Geometry: final body of the model. Coordinates: model frame, mm. A direction names the side the tool comes from. Give positions to 0.01 mm unless a question says otherwise; leave off trailing zeros. Loops run counter-clockwise (first coordinate to the right, second up) from the corner with the lowest first, then second, coordinate; pieces in that order, holes last. Notation, with made-up numbers: (-23, 8.25) -> (4, 8.25) arc R11 cw to (4, 29.25) -> close; hole circle Ø3 at (-38, 7). An arc over 180 degrees is marked (long way). Answer in a Markdown table with one row per item. Add a question column.
1) Section query B-B (y = 4.5). Return the cut outline in (x, z), plus the area to 3 significant figures.
2) Line query: line 1 (Z direction, x = 272, y = 6.75); line 2 (Y direction, x = 129, z = 2.5). Output: solid intervals per line, ascending. Write a range as from..to.
3) Access query for faces 1 (the flat face through (192, 9, 0)), 2 (the flat face through (192, 0, 7)). Directions: +Z, -Z, +X, -X, +Y, -Y. A direction counts if a zero-diameter tool reaches every point of the face in a straight line with its end or side. Return the directions, or none.
4) Section query A-A (x = 66.5). Return the cut outline in (y, z), plus the area to 3 significant figures.
5) First-contact query: P1, Ø4, axis at x = 17.145, z = 6.096, coming from the +Y side; P2, Ø4.5, axis at x = 258.445, y = 9.398, coming from the +Z side. Flat tips, straight axial feed; report the tip coordinate or a pass-through.
```python
from build123d import *

# Parameters (mm, degrees)
SKETCH1_W                    = 389.89
SKETCH1_H                    = 15.24
BASE_FLANGE1_DEPTH           = 1.524
EDGE_FLANGE1_STRIP_W         = 6.4008
EDGE_FLANGE1_STRIP_H         = 1.524
EDGE_FLANGE1_STRIP_CUT_DEPTH = 389.89
EDGE_FLANGE1_DEPTH           = 389.89
SKETCH9_R                    = 2.032
CUT_EXTRUDE1_DEPTH           = 2.54
SKETCH10_R                   = 1.778
CUT_EXTRUDE2_DEPTH           = 2.54


# Sheet-metal steps are written as plain solids
with BuildPart() as part:
    # Sketch1 → Base-Flange1 (new body)
    with BuildSketch(Plane.XY):
        with Locations((194.945, 7.62)):
            Rectangle(SKETCH1_W, SKETCH1_H)
    extrude(amount=-BASE_FLANGE1_DEPTH)

    # Edge-Flange1 strip (across the edge) → Edge-Flange1 strip cut (cut)
    with BuildSketch(Plane.YZ):
        with Locations((-1.524, -0.762)):
            Rectangle(EDGE_FLANGE1_STRIP_W, EDGE_FLANGE1_STRIP_H)
    extrude(amount=EDGE_FLANGE1_STRIP_CUT_DEPTH, mode=Mode.SUBTRACT)

    # Edge-Flange1 section (across the edge) → Edge-Flange1 (add)
    with BuildSketch(Plane.YZ):
        with BuildLine():
            Line((0, 0.1524), (0, 13.716))
            Line((0, 13.716), (1.524, 13.716))
            Line((1.524, 13.716), (1.524, 0.1524))
            ThreePointArc((1.524, 0.1524), (1.568636927, 0.044636927), (1.6764, 0))
            Line((1.6764, 0), (1.6764, -1.524))
            ThreePointArc((1.6764, -1.524), (0.491006192, -1.032993808), (0, 0.1524))
        make_face()
    extrude(amount=EDGE_FLANGE1_DEPTH)

    # Sketch9 → Cut-Extrude1 (cut)
    with BuildSketch(Plane.XY):
        with Locations((4.445, 9.398)):
            Circle(SKETCH9_R)
        with Locations((131.445, 9.398)):
            Circle(SKETCH9_R)
        with Locations((258.445, 9.398)):
            Circle(SKETCH9_R)
        with Locations((385.445, 9.398)):
            Circle(SKETCH9_R)
    extrude(amount=-CUT_EXTRUDE1_DEPTH, mode=Mode.SUBTRACT)

    # Sketch10 → Cut-Extrude2 (cut)
    with BuildSketch(Plane(origin=(0, 1.524, 0), x_dir=(1, 0, 0), z_dir=(0, 1, 0))):
        with Locations(Location((372.745, -6.096, 0), (0, 0, 270))):
            Circle(SKETCH10_R)
        with Locations(Location((194.945, -6.096, 0), (0, 0, 270))):
            Circle(SKETCH10_R)
        with Locations(Location((17.145, -6.096, 0), (0, 0, 270))):
            Circle(SKETCH10_R)
    extrude(amount=-CUT_EXTRUDE2_DEPTH, mode=Mode.SUBTRACT)


solid = part.part
```
Evaluation:
| question | item | result |
|---|---|---|
| 1 | outline | (0, -1.52) -> (389.89, -1.52) -> (389.89, 0) -> (0, 0) -> close |
| 1 | area | 594 mm² |
| 2 | line 1 | -1.52..0 |
| 2 | line 2 | 0..1.52 |
| 3 | face 1 | +Z, +X, -X, +Y |
| 3 | face 2 | +Z, -Z, +X, -X, -Y |
| 4 | outline | (0, 0.15) arc R1.68 ccw to (1.68, -1.52) -> (15.24, -1.52) -> (15.24, 0) -> (1.68, 0) arc R0.15 cw to (1.52, 0.15) -> (1.52, 13.72) -> (0, 13.72) -> close |
| 4 | area | 43.5 mm² |
| 5 | P1 | y = 1.52 |
| 5 | P2 | z = 0 |
